Here's how the part is built. I have some questions about the finished solid (model axes, mm). Face numbers are marked on the shaded views. A direction names the side the tool comes from. Give positions to 0.01 mm unless a question says otherwise; leave off trailing zeros. Order: outer loops, then holes, each group sorted by start corner. A loop starts at its lowest first (then second) coordinate and runs counter-clockwise, first axis right, second up.
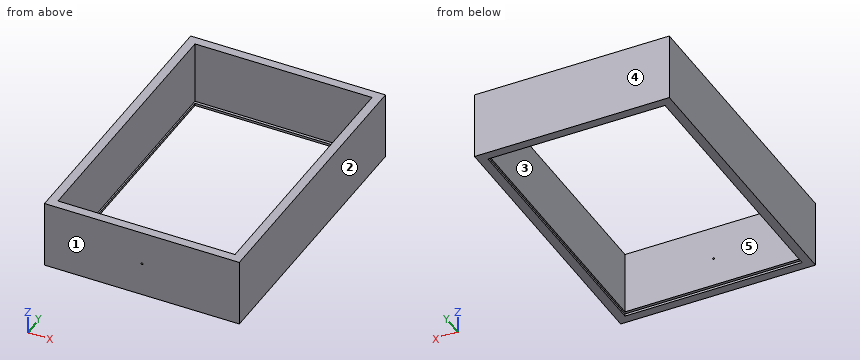
from build123d import *

# Parameters (mm, degrees)
F0_W      = 417
F0_H      = 145
F1_DEPTH  = 19
F3_DEPTH  = 590
F4_W      = 379
F4_H      = 5
F5_DEPTH  = 8
F6_W      = 19
F6_H      = 145
F7_DEPTH  = 379
F9_DEPTH  = 8
F11_DEPTH = 8
F13_DEPTH = 8
F14_R     = 2
F15_DEPTH = 19


with BuildPart() as f1:
    # F0 (on Front) → F1 (new body)
    with BuildSketch(Plane.XZ):
        with Locations((-15.645568, 27.064685)):
            Rectangle(F0_W, F0_H)
    extrude(amount=F1_DEPTH)

    # F2 (on face) → F3 (join)
    with BuildSketch(Plane.XZ.offset(19)):
        Polygon((-224.145568, 99.564685), (-224.145568, -45.435315), (-205.145568, -45.435315), (-205.145568, -40.435315), (-205.145568, -35.435315), (-205.145568, 99.564685), align=None)
        Polygon((173.854432, -40.435315), (173.854432, -45.435315), (192.854432, -45.435315), (192.854432, 99.564685), (173.854432, 99.564685), (173.854432, -35.435315), align=None)
    extrude(amount=F3_DEPTH)

    # F4 (on face) → F5 (cut)
    with BuildSketch(Plane.XZ.offset(19)):
        with Locations((-15.645568, -37.935315)):
            Rectangle(F4_W, F4_H)
    extrude(amount=-F5_DEPTH, mode=Mode.SUBTRACT)

    # F6 (on face) → F7 (join)
    with BuildSketch(Plane.YZ.offset(-205.145568)):
        with Locations((-599.5, 27.064685)):
            Rectangle(F6_W, F6_H)
    extrude(amount=F7_DEPTH)

    # F8 (on face) → F9 (cut)
    with BuildSketch(Plane(origin=(173.854432, 0, 0), x_dir=(0, -1, 0), z_dir=(-1, 0, 0))):
        Polygon((19, -35.435315), (11, -35.435315), (11, -40.435315), (19, -40.435315), (590, -40.435315), (590, -35.435315), align=None)
    extrude(amount=-F9_DEPTH, mode=Mode.SUBTRACT)

    # F10 (on face) → F11 (cut)
    with BuildSketch(Plane(origin=(0, -590, 0), x_dir=(-1, 0, 0), z_dir=(0, 1, 0))):
        Polygon((-173.854432, -35.435315), (-181.854432, -35.435315), (-181.854432, -40.435315), (-173.854432, -40.435315), (205.145568, -40.435315), (205.145568, -35.435315), align=None)
    extrude(amount=-F11_DEPTH, mode=Mode.SUBTRACT)

    # F12 (on face) → F13 (cut)
    with BuildSketch(Plane.YZ.offset(-205.145568)):
        Polygon((-590, -35.435315), (-598, -35.435315), (-598, -40.435315), (-590, -40.435315), (-19, -40.435315), (-11, -40.435315), (-11, -35.435315), (-19, -35.435315), align=None)
    extrude(amount=-F13_DEPTH, mode=Mode.SUBTRACT)

    # F14 (on face) → F15 (cut)
    with BuildSketch(Plane.XZ.offset(609)):
        with Locations((-15.645568, 27.064685)):
            Circle(F14_R)
    extrude(amount=-F15_DEPTH, mode=Mode.SUBTRACT)


solid = f1.part
Q1. For the marked faces 4 and 5, which set-ups out of +Z, -Z, +X, -X, +Y, -Y let a thin tool reach every point of the face, with its end or its side?
Filled sheet:
face 4: +Z, -Z, +X, -X, +Y
face 5: +Z, -Z
Q2. If we section it at C-C on y = -367.5: List the corners of the cut face in (x, z) for me.
Filled sheet:
outline: (-224.15, -45.44) - (-205.15, -45.44) - (-205.15, -40.44) - (-213.15, -40.44) - (-213.15, -35.44) - (-205.15, -35.44) - (-205.15, 99.56) - (-224.15, 99.56) - close; (173.85, -45.44) - (192.85, -45.44) - (192.85, 99.56) - (173.85, 99.56) - (173.85, -35.44) - (181.85, -35.44) - (181.85, -40.44) - (173.85, -40.44) - close
Q3. I'm going to push a flat-ended pin straight in: P1, Ø2.5, axis at x = -15.65, z = 27.06, coming from the -Y side. Where does the tip first touch, or does it pass through?
Filled sheet:
P1: stops at y = -19
Q4. I need wall thicknesses on L1, parallel to X at y = -24.5, z = 17; L2, parallel to Y at x = -135, z = 31.5; L3, parallel to Y at x = -83, z = -36. Which ranges of each line are inside material? Lowest first, please.
Filled sheet:
L1: x = -224.15 to -205.15, 173.85 to 192.85
L2: y = -609 to -590, -19 to 0
L3: y = -609 to -598, -11 to 0
Q5. Thinking about a two-plate mould opening in Y: for the marked faces 1, 2 and 3, which applies, released by +Y, released by -Y, zero draft, split by the parting line, or undercut?
Filled sheet:
face 1: released by -Y
face 2: zero draft
face 3: undercut
Q6. If we section it at B-B on z = 6.5: List the corners of the cut face in (x, y) for me.
Filled sheet:
outline: (-224.15, -609) - (192.85, -609) - (192.85, 0) - (-224.15, 0) - close; hole (-205.15, -590) - (173.85, -590) - (173.85, -19) - (-205.15, -19) - close
Q7. If we section it at A-A on x = 149: List the corners of the cut face in (y, z) for me, plus the area to 3 significant figures.
Filled sheet:
outline: (-609, -45.44) - (-590, -45.44) - (-590, -40.44) - (-598, -40.44) - (-598, -35.44) - (-590, -35.44) - (-590, 99.56) - (-609, 99.56) - close; (-19, -45.44) - (0, -45.44) - (0, 99.56) - (-19, 99.56) - (-19, -35.44) - (-11, -35.44) - (-11, -40.44) - (-19, -40.44) - close
area: 5,430 mm2
